Part model, mm, in its own coordinate system. Face numbers are marked on the shaded views. A direction names the side the tool comes from. Coordinates: 2 decimals unless noted, no trailing zeros. Loops run counter-clockwise (first coordinate to the right, second up) from the corner with the lowest first, then second, coordinate; pieces in that order, holes last. Notation, with made-up numbers: M 15.25,-7 L 27.25,-7 A37 ccw 27.25,29 Z; hole C -5.5,13 d6. An arc over 180 degrees is marked long. Answer as CSV lines item,"result". Start each with the question number.
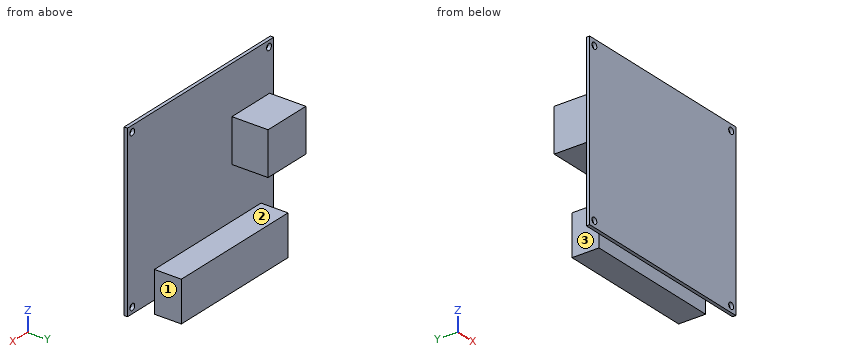
from build123d import *

# Parameters (mm, degrees)
SKETCH1_W           = 90
SKETCH1_H           = 80
SKETCH1_R           = 1.5
BOSS_EXTRUDE2_DEPTH = 1.6
SKETCH2_W           = 65.66
SKETCH2_H           = 19
BOSS_EXTRUDE3_DEPTH = 12.68
SKETCH3_W           = 23.240933929
SKETCH3_H           = 20.278854114
BOSS_EXTRUDE4_DEPTH = 17


with BuildPart() as part:
    # Sketch1 → Boss-Extrude2 (new body)
    with BuildSketch(Plane(origin=(0, 0, 0), x_dir=(1, 0, 0), z_dir=(0, 1, 0))):
        Rectangle(SKETCH1_W, SKETCH1_H)
        with Locations(Location((-42.1, 37.1, 0), (0, 0, 270))):
            Circle(SKETCH1_R, mode=Mode.SUBTRACT)
        with Locations(Location((42.1, 37.1, 0), (0, 0, 90))):
            Circle(SKETCH1_R, mode=Mode.SUBTRACT)
        with Locations(Location((-42.1, -37.1, 0), (0, 0, 90))):
            Circle(SKETCH1_R, mode=Mode.SUBTRACT)
        with Locations(Location((42.1, -37.1, 0), (0, 0, 270))):
            Circle(SKETCH1_R, mode=Mode.SUBTRACT)
    extrude(amount=BOSS_EXTRUDE2_DEPTH)

    # Sketch2 → Boss-Extrude3 (add)
    with BuildSketch(Plane(origin=(0, 1.6, 0), x_dir=(1, 0, 0), z_dir=(0, 1, 0))):
        with Locations((-4.35, 36.5)):
            Rectangle(SKETCH2_W, SKETCH2_H)
    extrude(amount=BOSS_EXTRUDE3_DEPTH)

    # Sketch3 → Boss-Extrude4 (add)
    with BuildSketch(Plane(origin=(0, 1.6, 0), x_dir=(1, 0, 0), z_dir=(0, 1, 0))):
        with Locations((-30.87398576, -7.2)):
            Rectangle(SKETCH3_W, SKETCH3_H)
    extrude(amount=BOSS_EXTRUDE4_DEPTH)


solid = part.part
Q1. Tool access for the marked faces 1, 2 and 3: list every direction of +Z, -Z, +X, -X, +Y, -Y with a clear straight run to the whole face (end or side of a thin tool).
Q2. Slice it at A-A, the plane z = -37.1. Write the cut outline in (x, y), and give its area (3 significant figures).
Q3. Wall check: L1, parallel to X at y = 0.4, z = -37.1; L2, parallel to Y at x = 32, z = 13; L3, parallel to Z at x = -24.5, y = 4.5. Give the ranges that are in metal, low to high.
Q4. Slice it at D-D, the plane z = 37.1. Write the cut outline in (x, y).
Q5. Flat gauge pins, fed straight in: P1, Ø1.8, axis at x = 42.1, z = -37.1, coming from the -Y side; P2, Ø21, axis at x = -19, z = -40.5, coming from the +Y side; P3, Ø2, axis at x = -33.5, y = 13, coming from the +Z side; P4, Ø3, axis at y = 13, z = 15.5, coming from the -X side. Where does each tip first touch, or does it go through?
Q6. Slice it at C-C, the plane x = 42.1. Write the cut outline in (y, z), and give its area (3 significant figures).
Q7. Slice it at B-B, the plane y = 3.5. Write the cut outline in (x, z), and give its area (3 significant figures).
Solved:
1,face 1,"+Z, -Z, +X, +Y"
1,face 2,"+X, -X, +Y"
1,face 3,"-Z, -X, +Y"
2,outline,"M -45,0 L -43.6,0 L -43.6,1.6 L -45,1.6 Z; M -40.6,0 L 40.6,0 L 40.6,1.6 L 28.48,1.6 L 28.48,14.28 L -37.18,14.28 L -37.18,1.6 L -40.6,1.6 Z; M 43.6,0 L 45,0 L 45,1.6 L 43.6,1.6 Z"
2,area,"967 mm2"
3,L1,"x = -45 to -43.6, -40.6 to 40.6, 43.6 to 45"
3,L2,"y = 0 to 1.6"
3,L3,"z = -46 to -27, -2.94 to 17.34"
4,outline,"M -45,0 L -43.6,0 L -43.6,1.6 L -45,1.6 Z; M -40.6,0 L 40.6,0 L 40.6,1.6 L -40.6,1.6 Z; M 43.6,0 L 45,0 L 45,1.6 L 43.6,1.6 Z"
5,P1,"passes through"
5,P2,"stops at y = 14.28"
5,P3,"stops at z = 17.34"
5,P4,"stops at x = -42.49"
6,outline,"M 0,-40 L 1.6,-40 L 1.6,-38.6 L 0,-38.6 Z; M 0,-35.6 L 1.6,-35.6 L 1.6,35.6 L 0,35.6 Z; M 0,38.6 L 1.6,38.6 L 1.6,40 L 0,40 Z"
6,area,"118 mm2"
7,outline,"M -42.49,-2.94 L -19.25,-2.94 L -19.25,17.34 L -42.49,17.34 Z; M -37.18,-46 L 28.48,-46 L 28.48,-27 L -37.18,-27 Z"
7,area,"1,720 mm2"
